```python
from build123d import *

# Parameters (mm, degrees)
EXTRUDE1_DEPTH = 10
SKETCH2_W      = 80
SKETCH2_H      = 100
EXTRUDE2_DEPTH = 50


with BuildPart() as part:
    # Sketch1 → Extrude1 (new body)
    with BuildSketch(Plane(origin=(0, 0, 0), x_dir=(0, 0, -1), z_dir=(1, 0, 0))):
        Polygon((0, 0), (357.360716499, 0), (357.360716499, 498.914273257), (347.360716499, 498.914273257), (347.360716499, 10), (0, 10), align=None)
    extrude(amount=EXTRUDE1_DEPTH)

    # Sketch2 → Extrude2 (add)
    with BuildSketch(Plane(origin=(0, 498.914273257, 0), x_dir=(-1, 0, 0), z_dir=(0, 1, 0))):
        with Locations((-5, -352.360716499)):
            Rectangle(SKETCH2_W, SKETCH2_H)
    extrude(amount=EXTRUDE2_DEPTH)


solid = part.part
```
The listing builds one solid part. Answer for the finished solid, in the listing's coordinates (mm). A direction names the side the tool comes from. Round coordinates to 2 decimals unless told otherwise and drop trailing zeros. Loops run counter-clockwise (first coordinate to the right, second up) from the corner with the lowest first, then second, coordinate; pieces in that order, holes last. Notation, with made-up numbers: (29, -40) - (34, -40) arc R25 ccw to (34, -8) - close; hole circle Ø7 at (27, -7.5). An arc over 180 degrees is marked (long way). Use one line per item in the form item = value. Start each with the question number.
1. The part is cut by section A-A on x = 23. Determine the outline of the cut face in (y, z), then the cut area to 3 significant figures.
2. Consider line 1 (Y direction, x = 2, z = -341.5); line 2 (Y direction, x = 3.5, z = -76.5); line 3 (Y direction, x = -8.5, z = -376.5). Determine where each line is inside the solid, lowest interval first. Write a range as [from, to].
3. The part is cut by section B-B on y = 515. Determine the outline of the cut face in (x, z).
4. Given pin 1 Ø3 at (x, y) = (4, 330.5) entering from +Z; pin 2 Ø8 at (x, z) = (-2, -227.5) entering from +Y; pin 3 Ø11 at (x, y) = (5, 300.5) entering from -Z, each flat-ended and moving along its own axis, determine where each tip first touches the part or whether it passes through.
5. A tool of negligible diameter and unlimited length cuts with its end or side. For faces 1 (the face through (0, 251, -350)), 2 (the face through (10, 251, -350)), 3 (the face through (-35, 524, -353)), from which of +Z, -Z, +X, -X, +Y, -Y can it reach the whole face along a straight path? Write none if from no direction.
Geometry check:
q1.outline = (498.91, -402.36) - (548.91, -402.36) - (548.91, -302.36) - (498.91, -302.36) - close
q1.area = 5,000 mm^2
q2.line_1 = [0, 10], [498.91, 548.91]
q2.line_2 = [0, 10]
q2.line_3 = [498.91, 548.91]
q3.outline = (-35, -402.36) - (45, -402.36) - (45, -302.36) - (-35, -302.36) - close
q4.pin_1 = -347.36
q4.pin_2 = 10
q4.pin_3 = -357.36
q5.face_1 = +Z, -Z, -X, -Y
q5.face_2 = +Z, -Z, +X, -Y
q5.face_3 = +Z, -Z, -X, +Y, -Y
